```python
from build123d import *

# Parameters (mm, degrees)
SKETCH_1_W          = 69.7
SKETCH_1_H          = 79.85
SKETCH_1_R          = 2.6
SKETCH_1_W_2        = 33.78
SKETCH_1_H_2        = 40.24
SKETCH_1_W_3        = 4
SKETCH_1_H_3        = 6.2
EXTRUDE_1_DEPTH     = 8.3
SKETCH_3_W          = 5.2
SKETCH_3_H          = 5.2
CUT_EXTRUDE_1_DEPTH = 10
SKETCH_5_W          = 5.2
SKETCH_5_H          = 5.2
CUT_EXTRUDE_2_DEPTH = 10


with BuildPart() as part:
    # Эскиз1 → Бобышка-Вытянуть1 (new body)
    with BuildSketch(Plane.XY):
        with Locations((-0.085003009, 0)):
            Rectangle(SKETCH_1_W, SKETCH_1_H)
        with Locations(Location((-27.697888562, 31.633987252, 0), (0, 0, 180))):
            Circle(SKETCH_1_R, mode=Mode.SUBTRACT)
        with Locations(Location((-27.697888562, -31.633987252, 0), (0, 0, 180))):
            Circle(SKETCH_1_R, mode=Mode.SUBTRACT)
        with Locations(Location((27.527882545, -31.633987252, 0), (0, 0, 180))):
            Circle(SKETCH_1_R, mode=Mode.SUBTRACT)
        with Locations(Location((27.527882545, 31.633987252, 0), (0, 0, 180))):
            Circle(SKETCH_1_R, mode=Mode.SUBTRACT)
        with Locations((-0.085003009, 0)):
            Rectangle(SKETCH_1_W_2, SKETCH_1_H_2, mode=Mode.SUBTRACT)
        with Locations((-27.697888562, 9.743987252)):
            Rectangle(SKETCH_1_W_3, SKETCH_1_H_3, mode=Mode.SUBTRACT)
        with Locations((27.527882545, 9.743987252)):
            Rectangle(SKETCH_1_W_3, SKETCH_1_H_3, mode=Mode.SUBTRACT)
    extrude(amount=EXTRUDE_1_DEPTH)

    # Эскиз3 → Вырез-Вытянуть1 (cut)
    with BuildSketch(Plane.XY.offset(8.3)):
        with Locations((-0.085003009, -31.733803261)):
            Rectangle(SKETCH_3_W, SKETCH_3_H)
    extrude(amount=-CUT_EXTRUDE_1_DEPTH, mode=Mode.SUBTRACT)

    # Эскиз5 → Вырез-Вытянуть2 (cut)
    with BuildSketch(Plane.XY.offset(8.3)):
        with Locations((-0.085003009, 31.633987252)):
            Rectangle(SKETCH_5_W, SKETCH_5_H)
    extrude(amount=-CUT_EXTRUDE_2_DEPTH, mode=Mode.SUBTRACT)


solid = part.part
```
Can you work these out from the model? Positions are in its coordinate system, mm. Coordinates: 2 decimals unless noted, no trailing zeros. Loops run counter-clockwise (first coordinate to the right, second up) from the corner with the lowest first, then second, coordinate; pieces in that order, holes last. Notation, with made-up numbers: M -15.5,15 L -3.5,15 A17 ccw -3.5,28 Z; hole C 20.25,-35 d7. An arc over 180 degrees is marked long. Put each result on its own line as item: value. Start each with the question number.
(1) We'd pull the mould along Y, two halves only. Please class faces 1 (the face through (-1, 39.925, 4)), 2 (the face through (-2.685, -32, 4)), 3 (the face through (-1, -39.925, 4)), 4 (the face through (0, -20.12, 4)): +Y half, -Y half, draft (parallel to the pull), parting line (faces both ways), or undercut.
(2) Imagine slicing it at A-A on y = 14. List the corners of the cut face in (x, z) for me (3 decimals), and give its area (3 significant figures).
(3) I need wall thicknesses on probe 1 along X at (y, z) = (-11, 1.75) (3 decimals); probe 2 along Y at (x, z) = (1, 5.75) (3 decimals); probe 3 along Y at (x, z) = (-3.5, 8.25) (3 decimals). Which ranges of each line are inside material? Lowest first, please.
(4) Imagine slicing it at C-C on x = -1. List the corners of the cut face in (y, z) for me (3 decimals), and give its area (3 significant figures).
(5) Imagine slicing it at B-B on x = -14. List the corners of the cut face in (y, z) for me (3 decimals), and give its area (3 significant figures).
(6) Will this pin go through, and if not, where does the flat tip stop? pin 1 Ø6 at (x, y) = (27.53, -31.63) entering from +Z.
(7) Imagine slicing it at D-D on z = 5.5. Give the number of separate pieces and of enclosed holes in the cut face, and give its area (3 significant figures).
Worked answers:
1. face 1: +Y half
1. face 2: undercut
1. face 3: -Y half
1. face 4: undercut
2. outline: M -34.935,0 L -16.975,0 L -16.975,8.3 L -34.935,8.3 Z; M 16.805,0 L 34.765,0 L 34.765,8.3 L 16.805,8.3 Z
2. area: 298 mm2
3. probe 1: x = -34.935 to -16.975, 16.805 to 34.765
3. probe 2: y = -39.925 to -34.334, -29.134 to -20.12, 20.12 to 29.034, 34.234 to 39.925
3. probe 3: y = -39.925 to -20.12, 20.12 to 39.925
4. outline: M -39.925,0 L -34.334,0 L -34.334,8.3 L -39.925,8.3 Z; M -29.134,0 L -20.12,0 L -20.12,8.3 L -29.134,8.3 Z; M 20.12,0 L 29.034,0 L 29.034,8.3 L 20.12,8.3 Z; M 34.234,0 L 39.925,0 L 39.925,8.3 L 34.234,8.3 Z
4. area: 242 mm2
5. outline: M -39.925,0 L -20.12,0 L -20.12,8.3 L -39.925,8.3 Z; M 20.12,0 L 39.925,0 L 39.925,8.3 L 20.12,8.3 Z
5. area: 329 mm2
6. pin 1: stops at z = 8.3
7. separate pieces: 1
7. enclosed holes: 9
7. area: 4,020 mm2
